from build123d import *

# Parameters (mm, degrees)
SKETCH1_W                               = 60
SKETCH1_H                               = 30
BOSS_EXTRUDE1_DEPTH                     = 9
SKETCH2_W                               = 60
SKETCH2_H                               = 9.7
BOSS_EXTRUDE2_DEPTH                     = 24
CHAMFER1_SIZE                           = 10
CSK_FOR_M4_SFHCS1_D                     = 4.5
CSK_FOR_M4_SFHCS1_DEPTH                 = 12
CSK_FOR_M4_SFHCS1_CSINK_D               = 8.96
CSK_FOR_M4_SFHCS1_CSINK_ANGLE           = 90
CSK_FOR_M4_SFHCS1_TIP                   = 1.351936393
CSK_FOR_M4_SFHCS3_D                     = 4.5
CSK_FOR_M4_SFHCS3_DEPTH                 = 12
CSK_FOR_M4_SFHCS3_CSINK_D               = 8.96
CSK_FOR_M4_SFHCS3_CSINK_ANGLE           = 90
CSK_FOR_M4_SFHCS3_TIP                   = 1.351936393
CBORE_FOR_M5_HEX_HEAD_BOLT2_D           = 4.5
CBORE_FOR_M5_HEX_HEAD_BOLT2_DEPTH       = 12
CBORE_FOR_M5_HEX_HEAD_BOLT2_CBORE_D     = 5
CBORE_FOR_M5_HEX_HEAD_BOLT2_CBORE_DEPTH = 4.2
CBORE_FOR_M5_HEX_HEAD_BOLT2_TIP         = 1.351936393
SKETCH9_W                               = 14.7
SKETCH9_H                               = 9.7
BOSS_EXTRUDE3_DEPTH                     = 10
CSK_FOR_M4_SFHCS2_D                     = 4.5
CSK_FOR_M4_SFHCS2_CSINK_D               = 8.96
CSK_FOR_M4_SFHCS2_CSINK_ANGLE           = 90
FILLET1_R                               = 5


with BuildPart() as part:
    # Sketch1 → Boss-Extrude1 (new body)
    with BuildSketch(Plane.XY):
        Rectangle(SKETCH1_W, SKETCH1_H)
    extrude(amount=BOSS_EXTRUDE1_DEPTH)

    # Sketch2 → Boss-Extrude2 (add)
    with BuildSketch(Plane.XY.offset(9)):
        with Locations((0, 10.15)):
            Rectangle(SKETCH2_W, SKETCH2_H)
        with Locations((0, -10.15)):
            Rectangle(SKETCH2_W, SKETCH2_H)
    extrude(amount=BOSS_EXTRUDE2_DEPTH)

    # Chamfer1
    chamfer1_edges = [part.edges().sort_by_distance(p)[0] for p in [
        (30, -10.15, 33),
        (-30, -10.15, 33),
    ]]
    chamfer(chamfer1_edges, length=CHAMFER1_SIZE)

    # CSK for M4 SFHCS1
    with Locations(Plane(origin=(0, -15, 0), x_dir=(-1, 0, 0), z_dir=(0, -1, 0))):
        with Locations((0, -28)):
            CounterSinkHole(CSK_FOR_M4_SFHCS1_D / 2, CSK_FOR_M4_SFHCS1_CSINK_D / 2, depth=CSK_FOR_M4_SFHCS1_DEPTH, counter_sink_angle=CSK_FOR_M4_SFHCS1_CSINK_ANGLE)
            with Locations((0, 0, -(CSK_FOR_M4_SFHCS1_DEPTH + CSK_FOR_M4_SFHCS1_TIP / 2))):  # 118° drill point
                Cone(0, CSK_FOR_M4_SFHCS1_D / 2, CSK_FOR_M4_SFHCS1_TIP, mode=Mode.SUBTRACT)

    # CSK for M4 SFHCS3
    with Locations(Plane(origin=(0, 15, 0), x_dir=(1, 0, 0), z_dir=(0, 1, 0))):
        with Locations((0, -28)):
            CounterSinkHole(CSK_FOR_M4_SFHCS3_D / 2, CSK_FOR_M4_SFHCS3_CSINK_D / 2, depth=CSK_FOR_M4_SFHCS3_DEPTH, counter_sink_angle=CSK_FOR_M4_SFHCS3_CSINK_ANGLE)
            with Locations((0, 0, -(CSK_FOR_M4_SFHCS3_DEPTH + CSK_FOR_M4_SFHCS3_TIP / 2))):  # 118° drill point
                Cone(0, CSK_FOR_M4_SFHCS3_D / 2, CSK_FOR_M4_SFHCS3_TIP, mode=Mode.SUBTRACT)

    # CBORE for M5 Hex Head Bolt2
    with Locations(Plane.XY.offset(9)):
        with Locations((-25, 0), (25, 0)):
            CounterBoreHole(CBORE_FOR_M5_HEX_HEAD_BOLT2_D / 2, CBORE_FOR_M5_HEX_HEAD_BOLT2_CBORE_D / 2, CBORE_FOR_M5_HEX_HEAD_BOLT2_CBORE_DEPTH, depth=CBORE_FOR_M5_HEX_HEAD_BOLT2_DEPTH)
            with Locations((0, 0, -(CBORE_FOR_M5_HEX_HEAD_BOLT2_DEPTH + CBORE_FOR_M5_HEX_HEAD_BOLT2_TIP / 2))):  # 118° drill point
                Cone(0, CBORE_FOR_M5_HEX_HEAD_BOLT2_D / 2, CBORE_FOR_M5_HEX_HEAD_BOLT2_TIP, mode=Mode.SUBTRACT)

    # Sketch9 → Boss-Extrude3 (add)
    with BuildSketch(Plane.XY.offset(33)):
        with Locations((-22.65, 10.15)):
            Rectangle(SKETCH9_W, SKETCH9_H)
    boss_extrude3 = extrude(amount=BOSS_EXTRUDE3_DEPTH)

    # CSK for M4 SFHCS2 (through all)
    with Locations(Plane.ZY.offset(30)):
        with Locations((38, 10)):
            csk_for_m4_sfhcs2 = CounterSinkHole(CSK_FOR_M4_SFHCS2_D / 2, CSK_FOR_M4_SFHCS2_CSINK_D / 2, counter_sink_angle=CSK_FOR_M4_SFHCS2_CSINK_ANGLE)

    # Mirror1: Boss-Extrude3, CSK for M4 SFHCS2 across plane
    add(boss_extrude3.mirror(Plane(origin=(0, 0, 0), x_dir=(0, 0, 1), z_dir=(1, 0, 0))))
    add(csk_for_m4_sfhcs2.mirror(Plane(origin=(0, 0, 0), x_dir=(0, 0, 1), z_dir=(1, 0, 0))), mode=Mode.SUBTRACT)

    # Fillet1
    # the kernel refuses this fillet: 5 mm, written as the material it takes off along each edge
    with BuildSketch(Plane(origin=(2.8, 5.3, 43), x_dir=(0, 0, -1), z_dir=(1, 0, 0)), Plane(origin=(42.5, 15, 43), x_dir=(0, 0, -1), z_dir=(-1, 0, 0))) as fillet1_piece_1:
        with BuildLine():
            CenterArc((FILLET1_R, FILLET1_R), FILLET1_R, 180, 90)
            Line((0, FILLET1_R), (0, 0))
            Line((0, 0), (FILLET1_R, 0))
        make_face()
    extrude(amount=39.7, mode=Mode.SUBTRACT)
    with BuildSketch(Plane(origin=(-2.8, 5.3, 43), x_dir=(0, 0, -1), z_dir=(-1, 0, 0)), Plane(origin=(-42.5, 15, 43), x_dir=(0, 0, -1), z_dir=(1, 0, 0))) as fillet1_piece_2:
        with BuildLine():
            CenterArc((FILLET1_R, -FILLET1_R), FILLET1_R, 90, 90)
            Line((0, -FILLET1_R), (0, 0))
            Line((0, 0), (FILLET1_R, 0))
        make_face()
    extrude(amount=39.7, mode=Mode.SUBTRACT)


solid = part.part
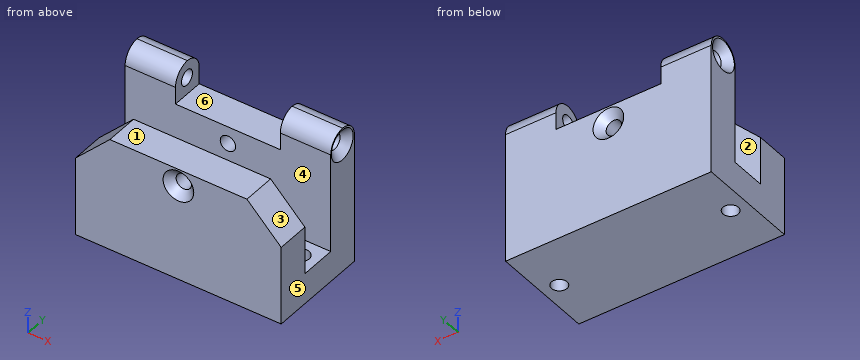
The model under review builds one solid part; all positions refer to its coordinate system, in mm. Face numbers are marked on the shaded views. A direction names the side the tool comes from. Coordinates: 2 decimals unless noted, no trailing zeros. Write each loop counter-clockwise with the first axis right and the second up, starting at its lowest first coordinate (ties: lowest second). Pieces come first, ordered by that corner, then holes. Notation, with made-up numbers: (16, 25) - (22, 25) arc R27 cw to (22, 42) - close; hole circle Ø10 at (60, 60). An arc over 180 degrees is marked (long way). Answer as a JSON object with one key per item and string values. Group by question number.
1. To check wall thickness, follow probe 1 along Y at (x, z) = (1.5, 14.5); probe 2 along Z at (x, y) = (0, 10.75); probe 3 along Y at (x, z) = (25, 6). State the ranges of each line that lie inside material, in increasing order.
2. Add section A-A (x = -25). Give the boundary of the cut face in (y, z), plus the area to 3 significant figures.
3. Mouldability with a two-part tool opening along X and no side actions: class the marked faces 4, 5 and 6 as pulls with the +X half, pulls with the -X half, needs draft (parallel to the pull), parting line crosses it, or undercut.
4. Add section D-D (z = 28). Give the boundary of the cut face in (x, y), plus the area to 3 significant figures.
5. Add section C-C (x = 18.5). Give the boundary of the cut face in (y, z), plus the area to 3 significant figures.
6. Machinability: for the marked faces 1, 2 and 3, which of the approach directions +Z, -Z, +X, -X, +Y, -Y give a long, thin tool a straight path to every point of the face, cutting with its end or side? Answer none if there is none.
7. Clearance check with flat-ended pins moving along their axes: pin 1 Ø1.5 at (x, y) = (6, 7) entering from +Z; pin 2 Ø1.5 at (x, y) = (-24.5, -1) entering from +Z; pin 3 Ø3 at (y, z) = (11.5, 40.5) entering from -X; pin 4 Ø8.5 at (x, y) = (9, 0) entering from +Z. State where each tip first meets the part, or that it passes through.
8. Add section B-B (y = -7). Give the boundary of the cut face in (x, z), plus the area to 3 significant figures.
Findings:
{
 "1": {"probe 1": "-15 to -5.3, 5.3 to 15", "probe 2": "0 to 25.75, 30.25 to 33", "probe 3": "-15 to -2.5, 2.5 to 15"},
 "2": {"outline": "(-15, 0) - (-2.25, 0) - (-2.25, 4.8) - (-2.5, 4.8) - (-2.5, 9) - (-5.3, 9) - (-5.3, 28) - (-15, 28) - close; (2.25, 0) - (15, 0) - (15, 38) arc R5 ccw to (10.15, 43) arc R5 ccw to (5.3, 38) - (5.3, 9) - (2.5, 9) - (2.5, 4.8) - (2.25, 4.8) - close; hole circle Ø4.5 at (10, 38)", "area": "715 mm²"},
 "3": {"face 4": "needs draft", "face 5": "pulls with the +X half", "face 6": "undercut"},
 "4": {"outline": "(-30, 5.3) - (-2.25, 5.3) - (-2.25, 12.77) - (-4.48, 15) - (-30, 15) - close; (-25, -15) - (-4.48, -15) - (-2.25, -12.77) - (-2.25, -5.3) - (-25, -5.3) - close; (2.25, -12.77) - (4.48, -15) - (25, -15) - (25, -5.3) - (2.25, -5.3) - close; (2.25, 5.3) - (30, 5.3) - (30, 15) - (4.48, 15) - (2.25, 12.77) - close", "area": "970 mm²"},
 "5": {"outline": "(-15, 0) - (15, 0) - (15, 38) arc R5 ccw to (10.15, 43) arc R5 ccw to (5.3, 38) - (5.3, 9) - (-5.3, 9) - (-5.3, 33) - (-15, 33) - close; hole circle Ø4.5 at (10, 38)", "area": "806 mm²"},
 "6": {"face 1": "+Z, +X, -X, -Y", "face 2": "+Z, +X, -X", "face 3": "+Z, +X, -Y"},
 "7": {"pin 1": "z = 33", "pin 2": "through", "pin 3": "x = -29.94", "pin 4": "z = 9"},
 "8": {"outline": "(-30, 0) - (30, 0) - (30, 23) - (20, 33) - (-20, 33) - (-30, 23) - close; hole circle Ø4.5 at (0, 28)", "area": "1,860 mm²"}
}
